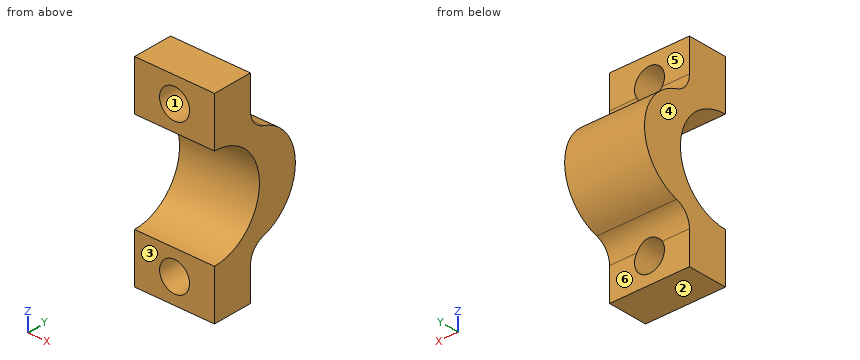
Autodesk Inventor part; units mm, degrees
ref_plane "YZ Plane" through (0, 0, 0) normal (1, 0, 0) x (0, 1, 0)
ref_plane "XZ Plane" through (0, 0, 0) normal (0, 1, 0) x (-1, 0, 0)
ref_plane "XY Plane" through (0, 0, 0) normal (0, 0, 1) x (1, 0, 0)
sketch "Skizze1" plane through (0, 0, 0) normal (1, 0, 0) x (0, 1, 0)
  line L0 (3.0012, 15.2548) -> (7.0012, 15.2548)
  line L1 (7.0012, -4.7452) -> (3.0012, -4.7452)
  arc A0 (3.0012, 0.2548) -> (3.0012, 10.2548) centre (3.0012, 5.2548) ccw
  arc A1 (7.0012, 0.2548) -> (7.0012, 10.2548) centre (7.0012, 5.2548) ccw
  line L2 (3.0012, -4.7452) -> (3.0012, 0.2548)
  line L3 (3.0012, 10.2548) -> (3.0012, 15.2548)
  line L4 (7.0012, 15.2548) -> (7.0012, 10.2548)
  line L5 (7.0012, 0.2548) -> (7.0012, -4.7452)
  point P0 (0, 0)
  dimension "d0" = 4
  dimension "d1" = 20
  dimension "d3" = 10
extrude "Extrusion1" add sketch "Skizze1" along normal blind 8
sketch "Skizze2" plane through (0, 7.0012, 15.2548) normal (0, 1, 0) x (1, 0, 0)
  line L0 (0, 0) -> (8, 0)
  line L1 (0, 20) -> (8, 20)
  line L2 (8, 20) -> (8, 15)
  line L3 (8, 5) -> (8, 0)
  point P0 (0, 15.2548)
  point P1 (4, 2.5)
  point P2 (4, 17.5)
  point P3 (4, 2.5)
  dimension "d6" = 2.5
  dimension "d7" = 2.5
  dimension "d8" = 4
  dimension "d9" = 4
hole "Bohrung1" at (4, 7.0012, 12.7548) at (4, 7.0012, -2.2452) direction (0, -1, 0) diameter 3 depth 8 tip angle 118
fillet "Rundung1" radius 2 2 edges at (4, 7.0012, 10.2548) (4, 7.0012, 0.2548)
properties part number "Klemme"
CAD build for the part. Positions are in the model's coordinates, mm. Face numbers are marked on the shaded views. A direction names the side the tool comes from. Round coordinates to 2 decimals unless told otherwise and drop trailing zeros. Loops run counter-clockwise (first coordinate to the right, second up) from the corner with the lowest first, then second, coordinate; pieces in that order, holes last. Notation, with made-up numbers: M -29.75,-3 L 15.25,-3 A21 cw 15.25,6 Z; hole C -28,-10 d10. An arc over 180 degrees is marked long. Use a Markdown table: item, result. Add a question column.
(1) Cut at B-B (x = 4). Give the cut face in (y, z), and give its area (3 significant figures).
(2) Which spindle directions (+Z, -Z, +X, -X, +Y, -Y) get a long thin tool onto all of the face, cutting with end or side? Do the marked faces 4, 5 and 6. Say none if no direction does.
(3) Cut at A-A (y = 4.75). Give the cut face in (x, z).
(4) Cut at C-C (z = 11.5). Give the cut face in (x, y).
(5) Flat gauge pins, fed straight in: pin 1 (4 mm diameter, centred on x = 2.5, z = 7, fed in from +Y); pin 2 (1 mm diameter, centred on x = 3.5, z = -3.5, fed in from +Y). Where does each tip first touch, or does it go through?
(6) Drill centre lines: line 1 (Z direction, x = 4.5, y = 5.5); line 2 (Z direction, x = 3, y = 5.5); line 3 (Z direction, x = 5.75, y = 6.5). Where is each one in solid material? Low to high.
(7) Cut at D-D (x = 1.75). Give the cut face in (y, z), and give its area (3 significant figures).
(8) Pull direction Z, two halves, no side cores. Call the marked faces 1, 2 and 3: +Z half, -Z half, draft (parallel to the pull), parting line (faces both ways), or undercut.
Geometry says:
| question | item | result |
|---|---|---|
| 1 | outline | M 3,-4.75 L 7,-4.75 L 7,-3.75 L 3,-3.75 Z; M 3,-0.75 L 7.13,-0.75 A2 cw 8.43,0.46 A5 ccw 8.43,10.05 A2 cw 7.13,11.25 L 3,11.25 L 3,10.25 A5 cw 3,0.25 Z; M 3,14.25 L 7,14.25 L 7,15.25 L 3,15.25 Z |
| 1 | area | 57.0 mm² |
| 2 | face 4 | +Z, -Z, -X, +Y, -Y |
| 2 | face 5 | +Z, +X, -X, +Y |
| 2 | face 6 | -Z, +X, -X, +Y |
| 3 | outline | M 0,-4.75 L 8,-4.75 L 8,0.57 L 0,0.57 Z; M 0,9.94 L 8,9.94 L 8,15.25 L 0,15.25 Z; hole C 4,-2.25 d3; hole C 4,12.75 d3 |
| 4 | outline | M 0,3 L 3.18,3 L 3.18,7.06 L 0,7.06 Z; M 4.82,3 L 8,3 L 8,7.06 L 4.82,7.06 Z |
| 5 | pin 1 | stops at y = 12 |
| 5 | pin 2 | stops at y = 7 |
| 6 | line 1 | z = -4.75 to -3.66, -0.83 to 0.92, 9.59 to 11.34, 14.17 to 15.25 |
| 6 | line 2 | z = -4.75 to -3.36, -1.13 to 0.92, 9.59 to 11.64, 13.87 to 15.25 |
| 6 | line 3 | z = -4.75 to 1.68, 8.83 to 15.25 |
| 7 | outline | M 3,-4.75 L 7,-4.75 L 7,-1.45 A2 cw 8.43,0.46 A5 ccw 8.43,10.05 A2 cw 7,11.96 L 7,15.25 L 3,15.25 L 3,10.25 A5 cw 3,0.25 Z |
| 7 | area | 81.0 mm² |
| 8 | face 1 | undercut |
| 8 | face 2 | -Z half |
| 8 | face 3 | draft |
